Build history of the part. All positions in model axes, mm. Face numbers are marked on the shaded views. A direction names the side the tool comes from. Round coordinates to 2 decimals unless told otherwise and drop trailing zeros. Order: outer loops, then holes, each group sorted by start corner. A loop starts at its lowest first (then second) coordinate and runs counter-clockwise, first axis right, second up. Notation, with made-up numbers: M 73,-7 L 89,-7 A10 ccw 89,7 Z; hole C 83.5,75.5 d4. An arc over 180 degrees is marked long. One line per item, written item: value. Start each with the question number.
Item 1: Tool access for the marked faces 1, 2 and 3: list every direction of +Z, -Z, +X, -X, +Y, -Y with a clear straight run to the whole face (end or side of a thin tool).
Item 2: Band-saw the part on B-B, the plane z = -192.5. Write the cut outline in (x, y), then the cut area to 3 significant figures.
Item 3: Band-saw the part on A-A, the plane z = -24. Write the cut outline in (x, y), then the cut area to 3 significant figures.
Item 4: Probe L1, parallel to Y at x = -1, z = -136.5; L2, parallel to Y at x = 0.5, z = -21; L3, parallel to X at y = 1, z = -186.5. List the from-to ranges inside material, lowest first.
Item 5: Pin check, flat tips, straight feed: pin 1 (4 mm diameter, centred on x = 8.5, z = -26, fed in from -Y); pin 2 (4 mm diameter, centred on y = -4, z = -94, fed in from +X); pin 3 (6 mm diameter, centred on y = -7.5, z = -126.5, fed in from +X). Stop position of each tip, or through.
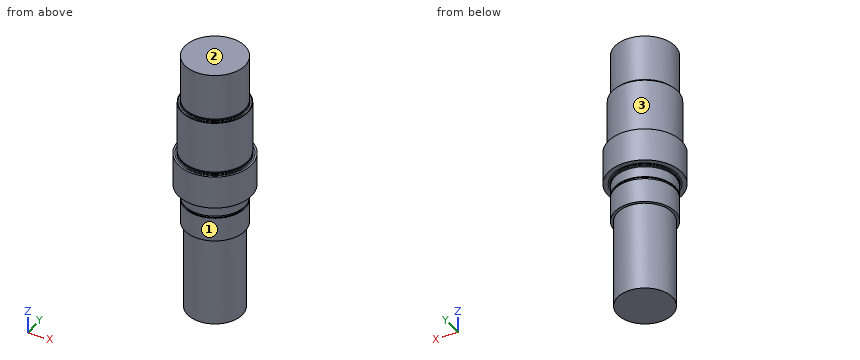
```python
from build123d import *

# Parameters (mm, degrees)
NUT_W = 2
NUT_H = 1


with BuildPart() as part:
    # Au_enkontur → Rotation_GK (revolve)
    with BuildSketch(Plane(origin=(0, 0, 0), x_dir=(0, 0, -1), z_dir=(1, 0, 0)), mode=Mode.PRIVATE) as rotation_gk_sk:
        Polygon((0, 0), (0, 27.5), (44.5, 27.5), (44.5, 30), (94, 30), (94, 33.5), (124, 33.5), (124, 27.5), (160, 27.5), (160, 25), (242, 25), (242, 0), align=None)
    revolve(rotation_gk_sk.sketch.rotate(Axis((0, 0, -88.99), (0, 0, 1)), 90), axis=Axis((0, 0, -88.99), (0, 0, 1)))  # turned: the seam where the file's is

    # Freistich 1 → Schnitt-Rotation_Freistich 1 (revolve, cut)
    with BuildSketch(Plane(origin=(0, 0, 0), x_dir=(0, 0, -1), z_dir=(1, 0, 0)), mode=Mode.PRIVATE) as schnitt_rotation_freistich_1_sk:
        with BuildLine():
            Line((42, 27.5), (43.043315314, 27.220444504))
            ThreePointArc((43.043315314, 27.220444504), (43.120291025, 27.205133083), (43.198606741, 27.2))
            Line((43.198606741, 27.2), (44.1, 27.2))
            ThreePointArc((44.1, 27.2), (44.552825748, 27.406364583), (44.694160841, 27.883503861))
            Line((44.694160841, 27.883503861), (44.5, 29.265030032))
            Line((44.5, 29.265030032), (42, 29.265030032))
            Line((42, 29.265030032), (42, 27.5))
        make_face()
    revolve(schnitt_rotation_freistich_1_sk.sketch.rotate(Axis((0, 0, -88.99), (0, 0, 1)), 90), axis=Axis((0, 0, -88.99), (0, 0, 1)), mode=Mode.SUBTRACT)  # turned: the seam where the file's is

    # Freistich 2 → Schnitt-Rotation_Freistich 2 (revolve, cut)
    with BuildSketch(Plane(origin=(0, 2.5, -49.5), x_dir=(0, 0, -1), z_dir=(1, 0, 0)), mode=Mode.PRIVATE) as schnitt_rotation_freistich_2_sk:
        with BuildLine():
            Line((42, 27.5), (43.043315314, 27.220444504))
            ThreePointArc((43.043315314, 27.220444504), (43.120291025, 27.205133083), (43.198606741, 27.2))
            Line((43.198606741, 27.2), (44.1, 27.2))
            ThreePointArc((44.1, 27.2), (44.552825748, 27.406364583), (44.694160841, 27.883503861))
            Line((44.694160841, 27.883503861), (44.5, 29.265030032))
            Line((44.5, 29.265030032), (42, 29.265030032))
            Line((42, 29.265030032), (42, 27.5))
        make_face()
    revolve(schnitt_rotation_freistich_2_sk.sketch.rotate(Axis((0, 0, -88.99), (0, 0, 1)), 90), axis=Axis((0, 0, -88.99), (0, 0, 1)), mode=Mode.SUBTRACT)  # turned: the seam where the file's is

    # Freistich 3 → Schnitt-Rotation_Freistich 3 (revolve, cut)
    with BuildSketch(Plane(origin=(0, 0, -168.5), x_dir=(0, 0, 1), z_dir=(-1, 0, 0)), mode=Mode.PRIVATE) as schnitt_rotation_freistich_3_sk:
        with BuildLine():
            Line((42, 27.5), (43.043315314, 27.220444504))
            ThreePointArc((43.043315314, 27.220444504), (43.120291025, 27.205133083), (43.198606741, 27.2))
            Line((43.198606741, 27.2), (44.1, 27.2))
            ThreePointArc((44.1, 27.2), (44.552825748, 27.406364583), (44.694160841, 27.883503861))
            Line((44.694160841, 27.883503861), (44.5, 29.265030032))
            Line((44.5, 29.265030032), (42, 29.265030032))
            Line((42, 29.265030032), (42, 27.5))
        make_face()
    revolve(schnitt_rotation_freistich_3_sk.sketch.rotate(Axis((0, 0, -88.99), (0, 0, 1)), 90), axis=Axis((0, 0, -88.99), (0, 0, 1)), mode=Mode.SUBTRACT)  # turned: the seam where the file's is

    # Nut → Schnitt-Rotation_Nut (revolve, cut)
    with BuildSketch(Plane(origin=(0, 0, 0), x_dir=(0, 0, -1), z_dir=(1, 0, 0)), mode=Mode.PRIVATE) as schnitt_rotation_nut_sk:
        with Locations((137, 27)):
            Rectangle(NUT_W, NUT_H)
    revolve(schnitt_rotation_nut_sk.sketch.rotate(Axis((0, 0, -88.99), (0, 0, 1)), 90), axis=Axis((0, 0, -88.99), (0, 0, 1)), mode=Mode.SUBTRACT)  # turned: the seam where the file's is


solid = part.part
```
Output:
1. face 1: -Z
1. face 2: +Z, +X, -X, +Y, -Y
1. face 3: +Z
2. outline: C 0,0 d50
2. area: 1,960 mm²
3. outline: C 0,0 d55
3. area: 2,380 mm²
4. L1: y = -26.48 to 26.48
4. L2: y = -27.5 to 27.5
4. L3: x = -24.98 to 24.98
5. pin 1: stops at y = -26.72
5. pin 2: stops at x = 33.44
5. pin 3: stops at x = 32.99
